from build123d import *

# Parameters (mm, degrees)
BOSS_EXTRUDE1_DEPTH  = 4.7625
M4_CLEARANCE_HOLE2_D = 4.5


with BuildPart() as part:
    # Sketch4 → Boss-Extrude1 (new body)
    with BuildSketch(Plane.XY.offset(-59.668926648)):
        with BuildLine():
            Line((5.401994847, 39.710959692), (-20.899520343, 39.710959692))
            ThreePointArc((-20.899520343, 39.710959692), (-22.812937505, 40.091562029), (-24.435054249, 41.175425786))
            Line((-24.435054249, 41.175425786), (-25.951045701, 42.691417238))
            ThreePointArc((-25.951045701, 42.691417238), (-33.729220295, 42.691417238), (-33.729220295, 34.913242645))
            Line((-33.729220295, 34.913242645), (-32.213228842, 33.397251193))
            ThreePointArc((-32.213228842, 33.397251193), (-31.129365086, 31.775134449), (-30.748762748, 29.861717287))
            Line((-30.748762748, 29.861717287), (-30.748762748, -6.439797903))
            ThreePointArc((-30.748762748, -6.439797903), (-31.129365086, -8.353215065), (-32.213228842, -9.975331809))
            Line((-32.213228842, -9.975331809), (-33.729220295, -11.491323262))
            ThreePointArc((-33.729220295, -11.491323262), (-33.729220295, -19.269497855), (-25.951045701, -19.269497855))
            Line((-25.951045701, -19.269497855), (-24.435054249, -17.753506402))
            ThreePointArc((-24.435054249, -17.753506402), (-22.812937505, -16.669642646), (-20.899520343, -16.289040308))
            Line((-20.899520343, -16.289040308), (5.401994847, -16.289040308))
            ThreePointArc((5.401994847, -16.289040308), (7.315412009, -16.669642646), (8.937528753, -17.753506402))
            Line((8.937528753, -17.753506402), (10.453520205, -19.269497855))
            ThreePointArc((10.453520205, -19.269497855), (18.231694798, -19.269497855), (18.231694798, -11.491323262))
            Line((18.231694798, -11.491323262), (16.715703346, -9.975331809))
            ThreePointArc((16.715703346, -9.975331809), (15.631839589, -8.353215065), (15.251237252, -6.439797903))
            Line((15.251237252, -6.439797903), (15.251237252, 29.861717287))
            ThreePointArc((15.251237252, 29.861717287), (15.631839589, 31.775134449), (16.715703346, 33.397251193))
            Line((16.715703346, 33.397251193), (18.231694798, 34.913242645))
            ThreePointArc((18.231694798, 34.913242645), (18.231694798, 42.691417238), (10.453520205, 42.691417238))
            Line((10.453520205, 42.691417238), (8.937528753, 41.175425786))
            ThreePointArc((8.937528753, 41.175425786), (7.315412009, 40.091562029), (5.401994847, 39.710959692))
        make_face()
        with BuildLine():
            Line((-6.148762748, 22.84660067), (-6.148762748, 24.460959692))
            Line((-6.148762748, 24.460959692), (-9.348762748, 24.460959692))
            Line((-9.348762748, 24.460959692), (-9.348762748, 22.84660067))
            ThreePointArc((-9.348762748, 22.84660067), (-7.748762748, 0.460959692), (-6.148762748, 22.84660067))
        make_face(mode=Mode.SUBTRACT)
    extrude(amount=BOSS_EXTRUDE1_DEPTH)

    # M4 Clearance Hole2 (through all)
    with Locations(Plane.XY.offset(-54.906426648)):
        with Locations((-29.840132998, 38.802329941), (14.342607502, 38.802329941), (14.342607502, -15.380410558), (-29.840132998, -15.380410558)):
            Hole(M4_CLEARANCE_HOLE2_D / 2)


solid = part.part
Geometry check sheet. Reference: the model listing, model coordinates, mm. A direction names the side the tool comes from. Give positions to 0.01 mm unless a question says otherwise; leave off trailing zeros. Loops run counter-clockwise (first coordinate to the right, second up) from the corner with the lowest first, then second, coordinate; pieces in that order, holes last. Notation, with made-up numbers: M -24,57 L -17,57 A36 ccw -17,94 Z; hole C 35,-32.5 d9. An arc over 180 degrees is marked long. Write each question's results on one line, items separated by ' | '.
1) Section check A-A, the plane x = 0. Record the boundary of the cut face in (y, z).
Answers follow:
outline: M -16.29,-59.67 L 3.56,-59.67 L 3.56,-54.91 L -16.29,-54.91 Z; M 19.87,-59.67 L 39.71,-59.67 L 39.71,-54.91 L 19.87,-54.91 Z
2) Thickness scan on line 1 (X direction, y = -17, z = -58.65); line 2 (X direction, y = 37.5, z = -55.9); line 3 (Y direction, x = 14, z = -56.8). Record the ranges inside material, lowest first.
Answers follow:
line 1: -35.1 to -31.4, -28.28 to -23.47, 7.97 to 12.78, 15.9 to 19.6 | line 2: -35.18 to -31.67, -28.01 to 12.51, 16.18 to 19.69 | line 3: -20.87 to -17.6, -13.16 to 36.58, 41.03 to 44.29
3) Gauge pin test, flat ends, axial feed: pin 1 (4 mm diameter, centred on x = -29.84, y = -15.38, fed in from +Z); pin 2 (6 mm diameter, centred on x = 14.34, y = -15.38, fed in from +Z); pin 3 (1 mm diameter, centred on x = -8, z = -57, fed in from -Y); pin 4 (2.5 mm diameter, centred on y = 11.5, z = -57.5, fed in from -X). Record the tip position at first contact, or that the pin passes through.
Answers follow:
pin 1: through | pin 2: z = -54.91 | pin 3: y = -16.29 | pin 4: x = -30.75
4) Section check D-D, the plane x = -29. Record the boundary of the cut face in (y, z).
Answers follow:
outline: M -20.82,-59.67 L -17.47,-59.67 L -17.47,-54.91 L -20.82,-54.91 Z; M -13.29,-59.67 L 36.72,-59.67 L 36.72,-54.91 L -13.29,-54.91 Z; M 40.89,-59.67 L 44.24,-59.67 L 44.24,-54.91 L 40.89,-54.91 Z
5) Release check for a two-part mould opening along X. For faces 4 (the face through (-27.592, -15.281, -57.321)), 5 (the face through (15.251, 11, -57)), 6 (the face through (-30.749, 12, -57)) record: +X half, -X half, draft (parallel to the pull), parting line (faces both ways), or undercut.
Answers follow:
face 4: undercut | face 5: +X half | face 6: -X half
6) Section check B-B, the plane z = -57.7. Count the separate pieces of the cut face and the enclosed holes in it, plus the area to 3 significant figures.
Answers follow:
separate pieces: 1 | enclosed holes: 5 | area: 2,370 mm2
7) Section check C-C, the plane y = 14.5. Record the boundary of the cut face in (x, z), plus the area to 3 significant figures.
Answers follow:
outline: M -30.75,-59.67 L -18.65,-59.67 L -18.65,-54.91 L -30.75,-54.91 Z; M 3.15,-59.67 L 15.25,-59.67 L 15.25,-54.91 L 3.15,-54.91 Z | area: 115 mm2
8) Tool access check on faces 1 (the face through (9.685, -18.501, -57.321)), 2 (the face through (-22.79, 40.08, -57.32)), 3 (the face through (17.48, -10.74, -57.32)). Record the directions out of +Z, -Z, +X, -X, +Y, -Y that give a thin tool (end or side, any length) a straight path to the whole face; none if there is none.
Answers follow:
face 1: +Z, -Z, -Y | face 2: +Z, -Z, +Y | face 3: +Z, -Z, +X
